Read the model definition and answer for the solid it produces. Units are mm, in the model's axes. Face numbers are marked on the shaded views. Round coordinates to 2 decimals unless told otherwise and drop trailing zeros. Order: outer loops, then holes, each group sorted by start corner. A loop starts at its lowest first (then second) coordinate and runs counter-clockwise, first axis right, second up. Notation, with made-up numbers: (-28, -3.5) -> (-15, -3.5) arc R33 cw to (-15, 30.5) -> close; hole circle Ø1 at (40.25, 41). An arc over 180 degrees is marked (long way). One line per item, written item: value. Start each with the question number.
1. A flat-ended cylindrical pin translates along its axis: pin 1 Ø2.5 at (x, y) = (8, 10.2) entering from +Z (3 decimals). Find the tip coordinate at first contact, or state that the pin passes through.
2. Section D-D (x = 14.25) is taken. Give the vertices of the cut face in (y, z).
3. Consider line 1 (Y direction, x = 8, z = 2.1); line 2 (X direction, y = 9, z = 4.45); line 3 (Y direction, x = 6.75, z = 3). Determine where each line is inside the solid, lowest interval first.
4. Section C-C (x = 9.75) is taken. Give the vertices of the cut face in (y, z), then the cut area to 3 significant figures.
5. Section B-B (y = 9.25) is taken. Give the vertices of the cut face in (x, z).
6. The mould has two halves that part along X. Classify the marked faces 1, 2 and 3: released by +X, released by -X, zero draft, split by the parting line, or undercut.
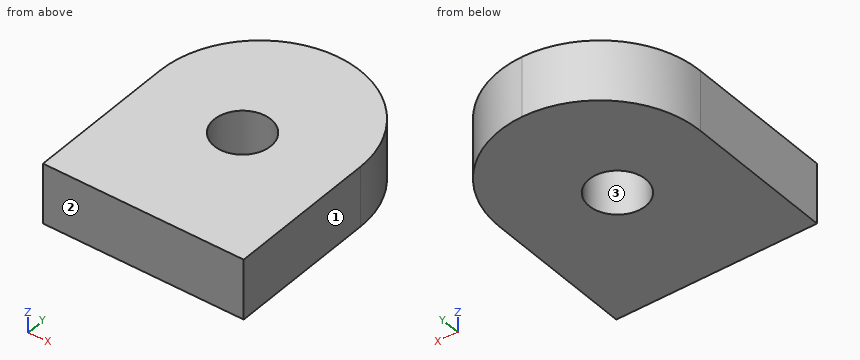
from build123d import *

# Parameters (mm, degrees)
SKETCH1_W           = 16
SKETCH1_H           = 20
BOSS_EXTRUDE1_DEPTH = 4.8
SKETCH2_R           = 2.25
CUT_EXTRUDE1_DEPTH  = 27.05839596
FILLET1_R           = 8


with BuildPart() as part:
    # Sketch1 → Boss-Extrude1 (new body)
    with BuildSketch(Plane.XY):
        with Locations((8, 10)):
            Rectangle(SKETCH1_W, SKETCH1_H)
    extrude(amount=BOSS_EXTRUDE1_DEPTH)

    # Sketch2 → Cut-Extrude1 (cut, through all)
    with BuildSketch(Plane.XY.offset(4.8)):
        with Locations((8, 10.2)):
            Circle(SKETCH2_R)
    extrude(amount=-CUT_EXTRUDE1_DEPTH, mode=Mode.SUBTRACT)

    # Fillet1
    fillet1_edges = [part.edges().sort_by_distance(p)[0] for p in [
        (16, 20, 2.4),
        (0, 20, 2.4),
    ]]
    fillet(fillet1_edges, radius=FILLET1_R - 0.0001)  # a hair under: the kernel refuses the full size


solid = part.part
Answer:
1. pin 1: through
2. outline: (0, 0) -> (16.99, 0) -> (16.99, 4.8) -> (0, 4.8) -> close
3. line 1: 0 to 7.95, 12.45 to 20
3. line 2: 0 to 6.1, 9.9 to 16
3. line 3: 0 to 8.33, 12.07 to 19.9
4. outline: (0, 0) -> (8.79, 0) -> (8.79, 4.8) -> (0, 4.8) -> close; (11.61, 0) -> (19.81, 0) -> (19.81, 4.8) -> (11.61, 4.8) -> close
4. area: 81.5 mm^2
5. outline: (0, 0) -> (5.96, 0) -> (5.96, 4.8) -> (0, 4.8) -> close; (10.04, 0) -> (16, 0) -> (16, 4.8) -> (10.04, 4.8) -> close
6. face 1: released by +X
6. face 2: zero draft
6. face 3: undercut
